Design review of the part built by this model. Coordinates are the model's own, in mm. A direction names the side the tool comes from. Coordinates: 2 decimals unless noted, no trailing zeros. Loops run counter-clockwise (first coordinate to the right, second up) from the corner with the lowest first, then second, coordinate; pieces in that order, holes last.
Q1. Machinability: for faces 1 (the face through (-23.95, 62.63, 2.46)), 2 (the face through (-2.733, -8.897, 2.465)), which of the approach directions +Z, -Z, +X, -X, +Y, -Y give a long, thin tool a straight path to every point of the face, cutting with its end or side? Answer none if there is none.
Q2. Add section C-C on x = 5. Give the boundary of the cut face in (y, z), and give its area (3 significant figures).
Q3. Add section D-D on z = 2.05. Give the number of separate pieces and of enclosed holes in the cut face, and give its area (3 significant figures).
Q4. Wall thickness on probe 1 along X at (y, z) = (25, 0.25); probe 2 along X at (y, z) = (30.5, 3.45); probe 3 along X at (y, z) = (-12, 4.3): over which ranges is each line inside the solid? List them lowest first.
Q5. Add section A-A on y = 40. Give the boundary of the cut face in (x, z), and give its area (3 significant figures).
Q6. Add section B-B on x = 22. Give the boundary of the cut face in (y, z), and give its area (3 significant figures).
Q7. For P1, Ø14.5, axis at x = 7.93, y = -14.39, coming from the +Z side; P2, Ø2, axis at x = -3.5, z = 2.5, coming from the -Y side; P3, Ø3, axis at x = -24.5, z = 3.5, coming from the -Y side, all flat-tipped, find the tip position at first contact; note any pin that passes through.
Q8. Draft analysis for pull direction Y (two halves, no side actions). For faces 3 (the face through (-27.37, 7.77, 2.46)), 4 (the face through (-8.37, 16.76, 2.46)), 5 (the face through (-15.58, -24.85, 2.46)), 6 (the face through (0.11, 69.12, 2.46)), state which applies: released by +Y, released by -Y, zero draft, split by the parting line, or undercut.
```python
from build123d import *

# Parameters (mm, degrees)
F0_R     = 4
F0_R_2   = 8
F1_DEPTH = 5


with BuildPart() as f1:
    # F0 (on Top) → F1 (new body)
    with BuildSketch(Plane.XY):
        with BuildLine():
            Line((19.390299, 73.280526), (-19.7102, 64.84542))
            ThreePointArc((-19.7102, 64.84542), (-24.001035, 62.582299), (-26.493853, 58.420709))
            Line((-26.493853, 58.420709), (-45.747654, -12.021702))
            ThreePointArc((-45.747654, -12.021702), (-44.398139, -19.613916), (-37.666102, -23.37458))
            Line((-37.666102, -23.37458), (7.133898, -26.367906))
            ThreePointArc((7.133898, -26.367906), (15.543966, -23.672904), (19.832321, -15.952653))
            Line((19.832321, -15.952653), (30.212015, 63.314377))
            ThreePointArc((30.212015, 63.314377), (27.385075, 71.103192), (19.390299, 73.280526))
        make_face()
        with Locations((-37.066102, -14.394603)):
            Circle(F0_R, mode=Mode.SUBTRACT)
        with BuildLine():
            ThreePointArc((-25.710896, -14.151075), (-27.402393, -13.486319), (-28.399698, -11.966962))
            ThreePointArc((-28.399698, -11.966962), (-28.586382, -11.37892), (-28.812914, -10.80505))
            ThreePointArc((-28.812914, -10.80505), (-29.0426, -9.269216), (-28.473597, -7.824301))
            Line((-28.473597, -7.824301), (-11.165939, 15.570463))
            ThreePointArc((-11.165939, 15.570463), (-8.325856, 16.755496), (-5.936497, 14.81608))
            Line((-5.936497, 14.81608), (0.396845, -2.512144))
            ThreePointArc((0.396845, -2.512144), (0.500674, -4.223675), (-0.349901, -5.712514))
            ThreePointArc((-0.349901, -5.712514), (-2.758659, -8.947656), (-3.959435, -12.798162))
            ThreePointArc((-3.959435, -12.798162), (-5.033997, -14.721694), (-7.132769, -15.392378))
            Line((-7.132769, -15.392378), (-25.710896, -14.151075))
        make_face(mode=Mode.SUBTRACT)
        with Locations((7.933898, -14.394603)):
            Circle(F0_R_2, mode=Mode.SUBTRACT)
        with BuildLine():
            ThreePointArc((-23.704846, 8.709998), (-27.426561, 7.795344), (-29.010443, 11.285196))
            Line((-29.010443, 11.285196), (-19.205892, 47.156357))
            ThreePointArc((-19.205892, 47.156357), (-18.590371, 47.707216), (-17.835441, 47.371966))
            Line((-17.835441, 47.371966), (-17.717148, 47.048311))
            Line((-17.717148, 47.048311), (-10.872426, 28.320938))
            ThreePointArc((-10.872426, 28.320938), (-10.720859, 26.862753), (-11.278377, 25.506859))
            Line((-11.278377, 25.506859), (-23.704846, 8.709998))
        make_face(mode=Mode.SUBTRACT)
        with Locations((-17.812301, 56.047808)):
            Circle(F0_R, mode=Mode.SUBTRACT)
        with BuildLine():
            ThreePointArc((11.860198, 0.185664), (10.79185, -1.741326), (8.695253, -2.41878))
            ThreePointArc((8.695253, -2.41878), (8.680991, -2.417881), (8.666727, -2.417))
            ThreePointArc((8.666727, -2.417), (7.056552, -1.827548), (6.032238, -0.452448))
            Line((6.032238, -0.452448), (-3.020297, 24.315573))
            ThreePointArc((-3.020297, 24.315573), (-3.171864, 25.773758), (-2.614346, 27.129653))
            Line((-2.614346, 27.129653), (15.979434, 52.262869))
            ThreePointArc((15.979434, 52.262869), (17.536186, 53.24565), (18.612615, 51.752118))
            Line((18.612615, 51.752118), (11.860198, 0.185664))
        make_face(mode=Mode.SUBTRACT)
        with BuildLine():
            Line((-6.542132, 57.456104), (10.439784, 61.119593))
            ThreePointArc((10.439784, 61.119593), (12.248976, 60.946714), (13.626362, 59.761021))
            ThreePointArc((13.626362, 59.761021), (13.726479, 59.602298), (13.829883, 59.445698))
            Line((13.829883, 59.445698), (-2.726784, 37.066048))
            ThreePointArc((-2.726784, 37.066048), (-5.566867, 35.881016), (-7.956226, 37.820432))
            Line((-7.956226, 37.820432), (-11.427107, 47.316869))
            ThreePointArc((-11.427107, 47.316869), (-11.564531, 48.863691), (-10.910133, 50.27199))
            ThreePointArc((-10.910133, 50.27199), (-9.565679, 52.443196), (-8.8852, 54.904627))
            ThreePointArc((-8.8852, 54.904627), (-8.119143, 56.552722), (-6.542132, 57.456104))
        make_face(mode=Mode.SUBTRACT)
        with Locations((21.288197, 64.482914)):
            Circle(F0_R, mode=Mode.SUBTRACT)
    extrude(amount=F1_DEPTH)


solid = f1.part
```
Entries:
1. face 1: +Z, -Z, -X, +Y
1. face 2: +Z, -Z
2. outline: (-26.23, 0) - (-21.84, 0) - (-21.84, 5) - (-26.23, 5) - close; (-6.95, 0) - (2.37, 0) - (2.37, 5) - (-6.95, 5) - close; (37.42, 0) - (47.51, 0) - (47.51, 5) - (37.42, 5) - close; (59.95, 0) - (70.18, 0) - (70.18, 5) - (59.95, 5) - close
2. area: 170 mm2
3. separate pieces: 1
3. enclosed holes: 8
3. area: 3,460 mm2
4. probe 1: x = -35.63 to -25.26, -11.65 to -3.18, 15.11 to 25.19
4. probe 2: x = -34.13 to -23.76, -11.67 to -0.12, 15.83 to 25.92
4. probe 3: x = -45.74 to -40.27, -33.86 to -28.39, -3.82 to 0.3, 15.57 to 20.35
5. outline: (-31.53, 0) - (-21.16, 0) - (-21.16, 5) - (-31.53, 5) - close; (-15.14, 0) - (-8.75, 0) - (-8.75, 5) - (-15.14, 5) - close; (-0.56, 0) - (6.91, 0) - (6.91, 5) - (-0.56, 5) - close; (17.07, 0) - (27.16, 0) - (27.16, 5) - (17.07, 5) - close
5. area: 172 mm2
6. outline: (0.6, 0) - (60.55, 0) - (60.55, 5) - (0.6, 5) - close; (68.42, 0) - (73.45, 0) - (73.45, 5) - (68.42, 5) - close
6. area: 325 mm2
7. P1: passes through
7. P2: stops at y = -25.72
7. P3: stops at y = -24.35
8. face 3: undercut
8. face 4: undercut
8. face 5: released by -Y
8. face 6: released by +Y
